Geometry check sheet. Reference: the model listing, model coordinates, mm. A direction names the side the tool comes from. Coordinates: 2 decimals unless noted, no trailing zeros. Loops run counter-clockwise (first coordinate to the right, second up) from the corner with the lowest first, then second, coordinate; pieces in that order, holes last. Notation, with made-up numbers: (58, 18) -> (64, 18) arc R16 cw to (64, 38) -> close; hole circle Ø9 at (24.5, 16). An arc over 180 degrees is marked (long way). Answer as a JSON object with one key per item and string values.
from build123d import *

# Parameters (mm, degrees)
BOSS_EXTRUDE1_DEPTH = 100
SKETCH2_R           = 2.2
SKETCH2_R_2         = 2
CUT_EXTRUDE2_DEPTH  = 6
SKETCH3_W           = 100
SKETCH3_H           = 8
BOSS_EXTRUDE2_DEPTH = 30
SKETCH4_W           = 100
SKETCH4_H           = 5
BOSS_EXTRUDE3_DEPTH = 30


with BuildPart() as part:
    # Sketch1 → Boss-Extrude1 (new body)
    with BuildSketch(Plane.XY):
        with BuildLine():
            Line((-57.167378994, 32.80487151), (-57.167378994, -17.19512849))
            Line((-57.167378994, -17.19512849), (37.112621006, -17.19512849))
            Line((37.112621006, -17.19512849), (37.112621006, 32.80487151))
            Line((37.112621006, 32.80487151), (17.112621006, 32.80487151))
            ThreePointArc((17.112621006, 32.80487151), (-10.027378994, 5.66487151), (-37.167378994, 32.80487151))
            Line((-37.167378994, 32.80487151), (-57.167378994, 32.80487151))
        make_face()
    extrude(amount=BOSS_EXTRUDE1_DEPTH)

    # Sketch2 → Cut-Extrude2 (cut)
    with BuildSketch(Plane(origin=(0, 32.80487151, 0), x_dir=(1, 0, 0), z_dir=(0, 1, 0))):
        with Locations(Location((-42.167378994, -5, 0), (0, 0, 270))):
            Circle(SKETCH2_R)
        with Locations(Location((-42.167378994, -15, 0), (0, 0, 270))):
            Circle(SKETCH2_R_2)
        with Locations(Location((-42.167378994, -25, 0), (0, 0, 270))):
            Circle(SKETCH2_R_2)
        with Locations(Location((-42.167378994, -35, 0), (0, 0, 270))):
            Circle(SKETCH2_R_2)
        with Locations(Location((-42.167378994, -45, 0), (0, 0, 270))):
            Circle(SKETCH2_R_2)
        with Locations(Location((-42.167378994, -55, 0), (0, 0, 270))):
            Circle(SKETCH2_R_2)
        with Locations(Location((-42.167378994, -65, 0), (0, 0, 270))):
            Circle(SKETCH2_R_2)
        with Locations(Location((-42.167378994, -75, 0), (0, 0, 270))):
            Circle(SKETCH2_R_2)
        with Locations(Location((-42.167378994, -85, 0), (0, 0, 270))):
            Circle(SKETCH2_R_2)
        with Locations(Location((22.112621006, -85, 0), (0, 0, 270))):
            Circle(SKETCH2_R_2)
        with Locations(Location((22.112621006, -75, 0), (0, 0, 90))):
            Circle(SKETCH2_R_2)
        with Locations(Location((22.112621006, -65, 0), (0, 0, 270))):
            Circle(SKETCH2_R_2)
        with Locations(Location((22.112621006, -55, 0), (0, 0, 90))):
            Circle(SKETCH2_R_2)
        with Locations(Location((22.112621006, -45, 0), (0, 0, 90))):
            Circle(SKETCH2_R_2)
        with Locations(Location((22.112621006, -35, 0), (0, 0, 270))):
            Circle(SKETCH2_R_2)
        with Locations(Location((22.112621006, -25, 0), (0, 0, 90))):
            Circle(SKETCH2_R_2)
        with Locations(Location((22.112621006, -15, 0), (0, 0, 90))):
            Circle(SKETCH2_R_2)
        with Locations(Location((22.112621006, -5, 0), (0, 0, 90))):
            Circle(SKETCH2_R)
    extrude(amount=-CUT_EXTRUDE2_DEPTH, mode=Mode.SUBTRACT)

    # Sketch3 → Boss-Extrude2 (add)
    with BuildSketch(Plane.ZY.offset(57.167378994)):
        with Locations((50, -13.19512849)):
            Rectangle(SKETCH3_W, SKETCH3_H)
    extrude(amount=BOSS_EXTRUDE2_DEPTH)

    # Sketch4 → Boss-Extrude3 (add)
    with BuildSketch(Plane(origin=(37.112621006, 0, 0), x_dir=(0, 0, -1), z_dir=(1, 0, 0))):
        with Locations((-50, -14.69512849)):
            Rectangle(SKETCH4_W, SKETCH4_H)
    extrude(amount=BOSS_EXTRUDE3_DEPTH)


solid = part.part
1. Section check A-A, the plane y = 17.5. Record the boundary of the cut face in (x, z), then the cut area to 3 significant figures.
Evaluation:
{"outline": "(-57.17, 0) -> (-32.44, 0) -> (-32.44, 100) -> (-57.17, 100) -> close; (12.39, 0) -> (37.11, 0) -> (37.11, 100) -> (12.39, 100) -> close", "area": "4,950 mm^2"}
2. Section check D-D, the plane y = 3. Record the boundary of the cut face in (x, z), then the cut area to 3 significant figures.
Evaluation:
{"outline": "(-57.17, 0) -> (37.11, 0) -> (37.11, 100) -> (-57.17, 100) -> close", "area": "9,430 mm^2"}
3. Section check C-C, the plane x = -70.5. Record the boundary of the cut face in (y, z), then the cut area to 3 significant figures.
Evaluation:
{"outline": "(-17.2, 0) -> (-9.2, 0) -> (-9.2, 100) -> (-17.2, 100) -> close", "area": "800 mm^2"}
4. Section check B-B, the plane z = 41. Record the boundary of the cut face in (x, y), then the cut area to 3 significant figures.
Evaluation:
{"outline": "(-87.17, -17.2) -> (67.11, -17.2) -> (67.11, -12.2) -> (37.11, -12.2) -> (37.11, 32.8) -> (17.11, 32.8) arc R27.14 cw to (-37.17, 32.8) -> (-57.17, 32.8) -> (-57.17, -9.2) -> (-87.17, -9.2) -> close", "area": "3,950 mm^2"}
5. Thickness scan on probe 1 along X at (y, z) = (31, 15); probe 2 along X at (y, z) = (29.7, 35); probe 3 along X at (y, z) = (16, 21.5). Record the ranges inside material, lowest first. Write a range as from..to.
Evaluation:
{"probe 1": "x = -57.17..-44.17, -40.17..-37.11, 17.05..20.11, 24.11..37.11", "probe 2": "x = -57.17..-44.17, -40.17..-36.99, 16.93..20.11, 24.11..37.11", "probe 3": "x = -57.17..-31.34, 11.28..37.11"}
6. Mould release check, pull along Z, two halves, no side actions. Record for faces 1 (the face through (-41.57, 29.85, 36.91)), 2 (the face through (-87.167, -13, 49)): released by +Z, released by -Z, zero draft, split by the parting line, or undercut.
Evaluation:
{"face 1": "undercut", "face 2": "zero draft"}
7. Depth check by flat-ended pin: P1, Ø3, axis at x = -42.17, z = 45, coming from the +Y side; P2, Ø2, axis at y = 22.5, z = 89.5, coming from the -X side; P3, Ø4, axis at y = -10, z = 79.5, coming from the +X side. Enter the tip coordinate at first touch or a pass-through.
Evaluation:
{"P1": "stops at y = 26.8", "P2": "stops at x = -57.17", "P3": "stops at x = 37.11"}
8. Tool access check on faces 3 (the face through (-72, -9.195, 49)), 4 (the face through (-40.184, 29.847, 64.74)), 5 (the face through (-47, 32.805, 49)). Record the directions out of +Z, -Z, +X, -X, +Y, -Y that give a thin tool (end or side, any length) a straight path to the whole face; none if there is none.
Evaluation:
{"face 3": "+Z, -Z, -X, +Y", "face 4": "+Y", "face 5": "+Z, -Z, +X, -X, +Y"}
